The model under review builds one solid part; all positions refer to its coordinate system, in mm. A direction names the side the tool comes from. Coordinates: 2 decimals unless noted, no trailing zeros. Write each loop counter-clockwise with the first axis right and the second up, starting at its lowest first coordinate (ties: lowest second). Pieces come first, ordered by that corner, then holes.
```python
from build123d import *

# Parameters (mm, degrees)
ESQUISSE1_W             = 5
ESQUISSE1_H             = 3
ESQUISSE1_W_2           = 3
ESQUISSE1_H_2           = 10
BOSS_EXTRU_1_DEPTH      = 3
ESQUISSE2_W             = 3
ESQUISSE2_H             = 3
ENL_V_MAT_EXTRU_1_DEPTH = 6


with BuildPart() as part:
    # Esquisse1 → Boss.-Extru.1 (new, symmetric)
    with BuildSketch(Plane.XY):
        with Locations((-12.5, 31.5)):
            Rectangle(ESQUISSE1_W, ESQUISSE1_H)
        with Locations((-2.5, 31.5)):
            Rectangle(ESQUISSE1_W, ESQUISSE1_H)
        with Locations((1.5, 25)):
            Rectangle(ESQUISSE1_W_2, ESQUISSE1_H_2)
        Polygon((-7, 15), (-7, 0), (0, 0), (0, 30), (-15, 30), (-15, 15), align=None)
        with Locations((1.5, 5)):
            Rectangle(ESQUISSE1_W_2, ESQUISSE1_H_2)
    extrude(amount=BOSS_EXTRU_1_DEPTH, both=True)

    # Esquisse2 → Enl_v. mat.-Extru.1 (cut)
    with BuildSketch(Plane.XY.offset(3)):
        with Locations((1.5, 28.5)):
            Rectangle(ESQUISSE2_W, ESQUISSE2_H)
    extrude(amount=-ENL_V_MAT_EXTRU_1_DEPTH, mode=Mode.SUBTRACT)


solid = part.part
```
Item 1: Mouldability with a two-part tool opening along X and no side actions: class faces 1 (the face through (1, 20, 0)), 2 (the face through (-5, 31, 0)), 3 (the face through (0, 30, 0)) as pulls with the +X half, pulls with the -X half, needs draft (parallel to the pull), parting line crosses it, or undercut.
Solved:
face 1: needs draft
face 2: undercut
face 3: pulls with the +X half
Item 2: For pin 1 (3.5 mm diameter, centred on y = 31.5, z = 1, fed in from +X); pin 2 (2 mm diameter, centred on x = -12, z = 1.5, fed in from -Y); pin 3 (1.5 mm diameter, centred on x = 1, z = -1.5, fed in from +Y); pin 4 (3.5 mm diameter, centred on x = 2, z = 0.5, fed in from -Y), all flat-tipped, find the tip position at first contact; note any pin that passes through.
Solved:
pin 1: stops at x = 0
pin 2: stops at y = 15
pin 3: stops at y = 27
pin 4: stops at y = 0
Item 3: Take a section at B-B, the plane y = 4.5. Write out the cut boundary in (x, z).
Solved:
outline: (-7, -3) - (3, -3) - (3, 3) - (-7, 3) - close
Item 4: Machinability: for faces 4 (the face through (-6, 17, -3)), 5 (the face through (1, 27, 0)), 6 (the face through (-10, 31, 0)), 7 (the face through (-7, 8, 0)), 8 (the face through (1, 10, 0)), which of the approach directions +Z, -Z, +X, -X, +Y, -Y give a long, thin tool a straight path to every point of the face, cutting with its end or side? Answer none if there is none.
Solved:
face 4: -Z, +X, -X, +Y, -Y
face 5: +Z, -Z, +X, +Y
face 6: +Z, -Z, +Y
face 7: +Z, -Z, -X, -Y
face 8: +Z, -Z, +X
Item 5: Take a section at C-C, the plane x = -11.75. Write out the cut boundary in (y, z), plus the area to 3 significant figures.
Solved:
outline: (15, -3) - (33, -3) - (33, 3) - (15, 3) - close
area: 108 mm2
Item 6: Take a section at A-A, the plane z = -2. Write out the cut boundary in (x, y).
Solved:
outline: (-15, 15) - (-7, 15) - (-7, 0) - (3, 0) - (3, 10) - (0, 10) - (0, 20) - (3, 20) - (3, 27) - (0, 27) - (0, 33) - (-5, 33) - (-5, 30) - (-10, 30) - (-10, 33) - (-15, 33) - close
Item 7: To check wall thickness, follow line 1 along Y through (x, z) = (2, 0.55); line 2 along X through (y, z) = (9, -1.35); line 3 along Y through (x, z) = (-12.5, -1.2). State the ranges of each line that lie inside material, in increasing order.
Solved:
line 1: y = 0 to 10, 20 to 27
line 2: x = -7 to 3
line 3: y = 15 to 33
